For this review, take the finished solid that the model builds, in its own axes (mm). A direction names the side the tool comes from. Coordinates: 2 decimals unless noted, no trailing zeros. Loops run counter-clockwise (first coordinate to the right, second up) from the corner with the lowest first, then second, coordinate; pieces in that order, holes last. Notation, with made-up numbers: (11.5, -16) - (44.5, -16) arc R24 cw to (44.5, 17) - close; hole circle Ø3 at (26.25, 73). An arc over 180 degrees is marked (long way). One line per item, written item: value. Start each with the question number.
1. Take a section at B-B, the plane x = 15. State the section outline as (y, z) points, and give its area (3 significant figures).
2. Take a section at D-D, the plane y = 12. State the section outline as (x, z) points, and give its area (3 significant figures).
3. Take a section at A-A, the plane z = 0. State the section outline as (x, y) points.
4. To check wall thickness, follow line 1 (Z direction, x = 28, y = 0); line 2 (Y direction, x = 4.5, z = -1.5); line 3 (Z direction, x = 19, y = -8). State the ranges of each line that lie inside material, in increasing order. Write a range as from..to.
5. For faces 4 (the face through (15.761, -1.464, 6.711)), 5 (the face through (12.52, -1.405, 9.982)), 6 (the face through (14.96, 0.97, -7.77)), list the 3-axis set-ups (+Z, -Z, +X, -X, +Y, -Y) from which the entire face can be reached by the end or side of a thin tool; tool diameter is ignored.
6. Insertion check: pin 1 (3 mm diameter, centred on x = 21, y = 3, fed in from -Z); pin 2 (5 mm diameter, centred on x = 6.5, y = -6.5, fed in from +Z); pin 3 (11.5 mm diameter, centred on y = 0, z = 0, fed in from -X); pin 4 (3 mm diameter, centred on y = 7.77, z = 5.51, fed in from +X). Each pin has a flat end and moves straight along its axis. Give the tip position at first contact, or say it passes through.
7. Take a section at C-C, the plane z = -9. State the section outline as (x, y) points.
8. The part is to be moulded in two halves that separate along X. For faces 1 (the face through (16.524, -0.632, 13.176)), 2 (the face through (0, 4, 4)), 3 (the face through (22, 2.85, 10)), say which applies: released by +X, released by -X, zero draft, split by the parting line, or undercut.
```python
from build123d import *

# Parameters (mm, degrees)
SKETCH1_R               = 15
BOSS_EXTRUDE1_DEPTH     = 29.5
SKETCH2_R               = 4.95
SKETCH2_R_2             = 1.7
CUT_EXTRUDE1_DEPTH      = 34
SKETCH3_R               = 1.65
CUT_EXTRUDE2_DEPTH      = 12
CUT_EXTRUDE3_DEPTH      = 1.3
CUT_EXTRUDE3_DEPTH_BACK = 1.3
SKETCH5_W               = 5.7
SKETCH5_H               = 2.6
CUT_EXTRUDE4_DEPTH      = 16


with BuildPart() as part:
    # Sketch1 → Boss-Extrude1 (new body)
    with BuildSketch(Plane.YZ):
        with Locations(Location((0, 0, 0), (0, 0, 270))):
            Circle(SKETCH1_R)
    extrude(amount=BOSS_EXTRUDE1_DEPTH)

    # Sketch2 → Cut-Extrude1 (cut)
    with BuildSketch(Plane.YZ.offset(29.5)):
        with Locations(Location((0, 0, 0), (0, 0, 270))):
            Circle(SKETCH2_R)
        with Locations(Location((-8.639482257, 3.974851738, 0), (0, 0, 270))):
            Circle(SKETCH2_R_2)
        with Locations(Location((7.768907949, 5.509495297, 0), (0, 0, 270))):
            Circle(SKETCH2_R_2)
        with Locations(Location((0.893753154, -9.467909236, 0), (0, 0, 270))):
            Circle(SKETCH2_R_2)
    extrude(amount=-CUT_EXTRUDE1_DEPTH, mode=Mode.SUBTRACT)

    # Sketch3 → Cut-Extrude2 (cut)
    with BuildSketch(Plane(origin=(0, 0, 15), x_dir=(0, 1, 0), z_dir=(0, 0, 1))):
        with Locations(Location((0, -15, 0), (0, 0, 270))):
            Circle(SKETCH3_R)
    extrude(amount=-CUT_EXTRUDE2_DEPTH, mode=Mode.SUBTRACT)

    # Sketch4 → Cut-Extrude3 (cut, two sides: drawn at the far end of the back side and taken through both)
    with BuildSketch(Plane(origin=(0, 0, 10), x_dir=(0, 1, 0), z_dir=(0, 0, 1)).offset(-CUT_EXTRUDE3_DEPTH_BACK)):
        Polygon((-2.85, -16.645448267), (0, -18.290896534), (2.85, -16.645448267), (2.85, -13.354551733), (0, -11.709103466), (-2.85, -13.354551733), align=None)
    extrude(amount=CUT_EXTRUDE3_DEPTH + CUT_EXTRUDE3_DEPTH_BACK, mode=Mode.SUBTRACT)

    # Sketch5 → Cut-Extrude4 (cut)
    with BuildSketch(Plane.YZ.offset(29.5)):
        with Locations((0, 10)):
            Rectangle(SKETCH5_W, SKETCH5_H)
    extrude(amount=-CUT_EXTRUDE4_DEPTH, mode=Mode.SUBTRACT)


solid = part.part
```
Solutions:
1. outline: (-2.85, 8.7) - (-2.85, 11.3) - (-1.65, 11.3) - (-1.65, 14.91) arc R15 ccw (long way) to (1.65, 14.91) - (1.65, 11.3) - (2.85, 11.3) - (2.85, 8.7) - (1.65, 8.7) - (1.65, 4.67) arc R4.95 cw (long way) to (-1.65, 4.67) - (-1.65, 8.7) - close; hole circle Ø3.4 at (-8.64, 3.97); hole circle Ø3.4 at (0.89, -9.47); hole circle Ø3.4 at (7.77, 5.51)
1. area: 563 mm2
2. outline: (0, -9) - (29.5, -9) - (29.5, 9) - (0, 9) - close
2. area: 531 mm2
3. outline: (0, -15) - (29.5, -15) - (29.5, -4.95) - (0, -4.95) - close; (0, 4.95) - (29.5, 4.95) - (29.5, 15) - (0, 15) - close
4. line 1: -15..-10.91, -8.02..-4.95, 4.95..8.7, 11.3..15
4. line 2: -14.92..-4.72, 4.72..14.92
4. line 3: -12.69..2.4, 5.55..12.69
5. face 4: +Z
5. face 5: +X
5. face 6: +X, -X
6. pin 1: z = -14.92
6. pin 2: z = 14.46
6. pin 3: x = 0
6. pin 4: through
7. outline: (0, -12) - (29.5, -12) - (29.5, -0.74) - (0, -0.74) - close; (0, 2.53) - (29.5, 2.53) - (29.5, 12) - (0, 12) - close
8. face 1: undercut
8. face 2: released by -X
8. face 3: zero draft
